Input: part model. Units: mm. Frame: model coordinates. A direction names the side the tool comes from. Coordinates: 2 decimals unless noted, no trailing zeros. Order: outer loops, then holes, each group sorted by start corner. A loop starts at its lowest first (then second) coordinate and runs counter-clockwise, first axis right, second up. Notation, with made-up numbers: (54, 50.25) - (84, 50.25) arc R18 ccw to (84, 60.25) - close; hole circle Ø4 at (-36.5, 0). An arc over 180 degrees is marked (long way). One line per question, with ' | ' between items.
Autodesk Inventor part; units mm, degrees
ref_plane "Work Plane2" through (5, 254.2, 0) normal (0, -1, 0) x (1, 0, 0)
ref_plane "Work Plane3" through (5, 144.2, 0) normal (0, -1, 0) x (1, 0, 0)
ref_plane "Work Plane4" through (0, 34.2, 0) normal (0, -1, 0) x (1, 0, 0)
sketch "Boceto1" plane through (0, 0, 0) normal (1, 0, 0) x (0, 1, 0)
  line L0 (0, 0) -> (330, 0)
  line L1 (330, 0) -> (330, -75)
  line L2 (330, -75) -> (0, -75)
  line L3 (0, -75) -> (0, 0)
  dimension "d0" = 330
  dimension "d1" = 75
extrude "Extrusión1" add sketch "Boceto1" along normal blind 5
sketch "Boceto2" plane through (5, 0, 0) normal (1, 0, 0) x (0, 0, -1)
  line L0 (75, 330) -> (0, 330)
  line L1 (75, 0) -> (75, 330)
  line L2 (0, 330) -> (75, 330)
  line L3 (75, 330) -> (75, 250)
  line L4 (75, 250) -> (0, 250)
  line L5 (0, 250) -> (0, 330)
  line L6 (75, 140) -> (0, 140)
  line L7 (0, 140) -> (0, 220)
  line L8 (0, 220) -> (75, 220)
  line L9 (75, 220) -> (75, 140)
  line L10 (75, 30) -> (0, 30)
  line L11 (0, 30) -> (0, 110)
  line L12 (0, 110) -> (75, 110)
  line L13 (75, 110) -> (75, 30)
  point P0 (0, 0)
  dimension "d4" = 80
  dimension "d7" = 110
extrude "Extrusión2" add sketch "Boceto2" along normal blind 4
sketch "Boceto3" plane through (0, 330, 0) normal (0, 1, 0) x (1, 0, 0)
  line L0 (7, 0) -> (4, 0)
  line L1 (4, 0) -> (4, 75)
  line L2 (4, 75) -> (7, 75)
  line L3 (7, 75) -> (7, 0)
  line L4 (0, 75) -> (0, 0)
  line L5 (9, 75) -> (9, 0)
  line L6 (0, 0) -> (9, 0)
  line L7 (0, 75) -> (9, 75)
  dimension "d14" = 4
  dimension "d15" = 2
  dimension "d16" = 0
  dimension "d17" = 0
  dimension "d62" = 3
sketch "Boceto8" plane through (5, 220, 0) normal (0, 1, 0) x (1, 0, 0)
  line L0 (-1, 0) -> (-1, 75)
  line L1 (2, 75) -> (2, 0)
  line L2 (-5, 0) -> (4, 0)
  line L3 (-5, 75) -> (4, 75)
sketch "Boceto9" plane through (5, 110, 0) normal (0, 1, 0) x (1, 0, 0)
  line L0 (2, 75) -> (2, 0)
  line L1 (-1, 0) -> (-1, 75)
  line L2 (-5, 0) -> (4, 0)
  line L3 (-5, 75) -> (4, 75)
extrude "Extrusión3" cut sketch "Boceto3" against normal blind 30 contours L0 L1 L2 L3
extrude "Extrusión4" cut sketch "Boceto8" against normal blind 30
extrude "Extrusión5" cut sketch "Boceto9" against normal blind 30
sketch "Boceto10" plane through (0, 0, 0) normal (-1, 0, 0) x (0, 0, 1)
  line L0 (-75, 0) -> (-75, 330)
  line L1 (-75, 330) -> (0, 330)
  line L2 (-75, 0) -> (-70, 0)
  line L3 (-70, 0) -> (-70, 330)
  line L4 (-70, 330) -> (-75, 330)
  line L5 (-75, 330) -> (-75, 0)
  point P0 (0, 0)
  dimension "d24" = 5
extrude "Extrusión6" add sketch "Boceto10" against normal blind 100
sketch "Boceto11" plane through (5, 0, -70) normal (0, 0, 1) x (1, 0, 0)
  line L0 (95, 330) -> (95, 0)
  line L1 (-5, 0) -> (95, 0)
  line L2 (95, 330) -> (90, 330)
  line L3 (90, 330) -> (90, 0)
  line L4 (90, 0) -> (95, 0)
  line L5 (95, 0) -> (95, 330)
  dimension "d27" = 5
extrude "Extrusión7" add sketch "Boceto11" along normal blind 70
sketch "Boceto12" plane through (95, 0, -70) normal (-1, 0, 0) x (0, 0, 1)
  line L0 (70, 0) -> (70, 330)
  line L1 (-5, 0) -> (-5, 330)
  line L2 (70, 250) -> (-5, 250)
  line L3 (-5, 250) -> (-5, 220)
  line L4 (-5, 220) -> (70, 220)
  line L5 (70, 220) -> (70, 250)
  line L6 (-5, 330) -> (70, 330)
  line L7 (70, 140) -> (-5, 140)
  line L8 (-5, 140) -> (-5, 110)
  line L9 (-5, 110) -> (70, 110)
  line L10 (70, 110) -> (70, 140)
  line L11 (70, 30) -> (-5, 30)
  line L12 (-5, 30) -> (-5, 0)
  line L13 (-5, 0) -> (70, 0)
  line L14 (70, 0) -> (70, 30)
  point P0 (70, 0)
  point P1 (70, 30)
  point P2 (-5, 30)
  point P3 (70, 140)
  point P4 (-5, 140)
  point P5 (-5, 250)
  dimension "d30" = 80
  dimension "d31" = 30
  dimension "d34" = 110
extrude "Extrusión8" add sketch "Boceto12" along normal blind 4 contours L13 L1 L11 L0 | L9 L1 L7 L0 | L4 L1 L2 L0
sketch "Boceto16" plane through (100, 0, 0) normal (1, 0, 0) x (0, 0, -1)
  line L0 (70, 250) -> (0, 250)
  line L1 (0, 330) -> (0, 250)
  line L2 (70, 330) -> (0, 330)
  line L3 (70, 250) -> (70, 330)
  line L4 (70, 140) -> (0, 140)
  line L5 (0, 220) -> (0, 140)
  line L6 (0, 220) -> (70, 220)
  line L7 (70, 140) -> (70, 220)
  line L8 (70, 30) -> (0, 30)
  line L9 (0, 110) -> (0, 30)
  line L10 (0, 110) -> (70, 110)
  line L11 (70, 30) -> (70, 110)
  point P0 (0, 0)
extrude "Extrusión12" cut sketch "Boceto16" against normal blind 10
sketch "Boceto25" plane through (0, 0, 0) normal (0, 0, 1) x (1, 0, 0)
  line L0 (7, 330) -> (7, 300) construction
  line L1 (7, 300) -> (7, 330) construction
  line L2 (7, 330) -> (125.2499, 220) construction
  line L3 (7, 330) -> (9, 328.1395)
  line L4 (9, 330) -> (9, 250)
  line L5 (7, 330) -> (9, 330)
  line L6 (8, 330) -> (7, 330)
  line L7 (7, 220) -> (9, 220)
  line L8 (7, 220) -> (9, 218.1395)
  line L9 (9, 220) -> (9, 140)
  line L10 (7, 220) -> (9.7315, 220) construction
  line L11 (9, 218.1395) -> (9, 220)
  line L12 (9, 220) -> (7, 220)
  line L13 (7, 110) -> (9, 110)
  line L14 (7, 110) -> (9, 108.1395)
  line L15 (9, 108.1395) -> (9, 110)
  line L16 (9, 110) -> (7, 110)
  point P0 (0, 0)
  dimension "d57" = 42.93
  dimension "d106" = 42.93
extrude "Extrusión13" cut sketch "Boceto25" against normal blind 70
sketch "Boceto26" plane through (5, 0, 0) normal (1, 0, 0) x (0, 0, -1)
  line L0 (70, 0) -> (70, 30)
  line L1 (70, 30) -> (0, 30)
  line L2 (0, 30) -> (0, 0)
  line L3 (0, 0) -> (70, 0)
extrude "Extrusión14" cut sketch "Boceto26" against normal blind 10
sketch "Boceto27" plane through (91, 220, -70) normal (0, -1, 0) x (1, 0, 0)
  line L0 (0, 0) -> (0, 70) construction
  line L1 (0, 70) -> (-37.4235, 70) construction
  circle A0 centre (-7.5, 70) radius 7.5
  line L2 (0, 50) -> (-7.5, 50)
  line L3 (-7.5, 50) -> (-7.5, 70)
  line L4 (-7.5, 70) -> (0, 70)
  line L5 (0, 70) -> (0, 50)
  circle A1 centre (-7.5, 70) radius 4
  point P0 (-91, 70)
  point P1 (-7.5, 62.5)
  dimension "d64" = 15
  dimension "d63" = 20
  dimension "d65" = 8
sketch "Boceto28" plane through (91, 110, -70) normal (0, -1, 0) x (1, 0, 0)
  line L0 (0, 50) -> (-7.5, 50)
  line L1 (-7.5, 50) -> (-7.5, 70)
  circle A0 centre (-7.5, 70) radius 7.5
  circle A1 centre (-7.5, 70) radius 4
  line L2 (0, 70) -> (-37.4235, 70) construction
  line L3 (0, 70) -> (0, 50)
  point P0 (-91, 70)
  point P1 (-7.5, 62.5)
sketch "Boceto29" plane through (0, 0, -75) normal (0, -1, 0) x (1, 0, 0)
  line L0 (91, 55) -> (83.5, 55)
  line L1 (83.5, 55) -> (83.5, 75)
  circle A0 centre (83.5, 75) radius 7.5
  circle A1 centre (83.5, 75) radius 4
  line L2 (83.5, 75) -> (91, 75)
  line L3 (91, 75) -> (91, 55)
  point P0 (0, 75)
  point P1 (83.5, 67.5)
extrude "Extrusión15" add sketch "Boceto27" against normal blind 8.4 contours L4 A1 L3 A0 | L5 L2 L3 A0 | A0 L3 A1 L4
extrude "Extrusión16" add sketch "Boceto28" against normal blind 8.4
extrude "Extrusión17" add sketch "Boceto29" against normal blind 8.4 contours L0 L1 A0 L3 | L2 A1 L1 A0 | A0 L1 A1 L2
sketch "Boceto30" plane through (91, 220, -70) normal (0, -1, 0) x (1, 0, 0)
  circle A0 centre (-7.5, 70) radius 4
  line L0 (0, 0) -> (-91, 0)
  line L1 (-91, 0) -> (-91, -5)
  line L2 (-91, -5) -> (9, -5)
  line L3 (9, -5) -> (9, 70)
  line L4 (9, 70) -> (0, 70)
  arc A1 (0, 70) -> (-7.5, 62.5) centre (-7.5, 70) ccw
  line L5 (-7.5, 62.5) -> (-7.5, 50)
  line L6 (-7.5, 50) -> (0, 50)
  line L7 (0, 0) -> (0, 50)
  line L8 (0, 50) -> (0, 70)
  point P0 (-91, 70)
sketch "Boceto31" plane through (91, 110, -70) normal (0, -1, 0) x (1, 0, 0)
  line L0 (0, 50) -> (0, 70)
  circle A0 centre (-7.5, 70) radius 4
  line L1 (9, 0) -> (0, 0)
  line L2 (9, 70) -> (9, 0)
  line L3 (0, 70) -> (9, 70)
  arc A1 (0, 70) -> (-7.5, 62.5) centre (-7.5, 70) ccw
  line L4 (-7.5, 62.5) -> (-7.5, 50)
  line L5 (-7.5, 50) -> (0, 50)
  line L6 (0, 0) -> (0, 50)
  point P0 (-91, 70)
sketch "Boceto32" plane through (0, 0, -75) normal (0, -1, 0) x (1, 0, 0)
  circle A0 centre (83.5, 75) radius 4
  line L0 (100, 5) -> (91, 5)
  line L1 (100, 75) -> (100, 5)
  line L2 (91, 75) -> (100, 75)
  arc A1 (91, 75) -> (83.5, 67.5) centre (83.5, 75) ccw
  line L3 (83.5, 67.5) -> (83.5, 55)
  line L4 (83.5, 55) -> (91, 55)
  line L5 (91, 5) -> (91, 55)
  line L6 (91, 55) -> (91, 75)
  point P0 (0, 75)
extrude "Extrusión18" cut sketch "Boceto32" against normal blind 4.2 contours L4 L3 A1 L6
extrude "Extrusión19" cut sketch "Boceto31" against normal blind 4.2 contours L5 L4 A1 L0
extrude "Extrusión20" cut sketch "Boceto30" against normal blind 4.2 contours L6 L5 A1 L8
thread "Rosca1"
ref_plane "Work Plane2" through (5, 254.2, 0) normal (0, -1, 0) x (1, 0, 0)
sketch "Sketch33" plane through (5, 254.2, 0) normal (0, -1, 0) x (1, 0, 0)
  line L0 (4, 0) -> (4, -20)
  line L1 (4, -20) -> (11.5, -20)
  line L2 (11.5, -20) -> (11.5, 0)
  line L3 (11.5, 0) -> (4, 0)
  circle A0 centre (11.5, 0) radius 4
  circle A1 centre (11.5, 0) radius 7.5
  point P0 (-5, 0)
  point P1 (4, 0)
  point P2 (11.5, -7.5)
  dimension "d81" = 20
  dimension "d82" = 7.5
  dimension "d83" = 20
  dimension "d84" = 8
  dimension "d85" = 15
extrude "Extrusion21" add sketch "Sketch33" against normal blind 4.2 contours A1 L2 L1 L0 | A1 L2 A0 L3 | L3 A0 L2 A1
ref_plane "Work Plane3" through (5, 144.2, 0) normal (0, -1, 0) x (1, 0, 0)
sketch "Sketch34" plane through (5, 144.2, 0) normal (0, -1, 0) x (1, 0, 0)
  line L0 (4, 0) -> (4, -20)
  line L1 (4, -20) -> (11.5, -20)
  line L2 (11.5, -20) -> (11.5, 0)
  line L3 (11.5, 0) -> (4, 0)
  circle A0 centre (11.5, 0) radius 4
  circle A1 centre (11.5, 0) radius 7.5
  point P0 (-5, 0)
  point P1 (11.5, -7.5)
  dimension "d89" = 20
  dimension "d90" = 7.5
  dimension "d91" = 20
  dimension "d92" = 8
  dimension "d93" = 15
extrude "Extrusion22" add sketch "Sketch34" against normal blind 4.2 contours A1 L2 L1 L0 | A1 L2 A0 L3 | L3 A0 L2 A1
ref_plane "Work Plane4" through (0, 34.2, 0) normal (0, -1, 0) x (1, 0, 0)
sketch "Sketch35" plane through (0, 34.2, 0) normal (0, -1, 0) x (1, 0, 0)
  line L0 (9, 0) -> (9, -20)
  line L1 (9, -20) -> (16.5, -20)
  line L2 (16.5, -20) -> (16.5, 0)
  line L3 (16.5, 0) -> (9, 0)
  circle A0 centre (16.5, 0) radius 4
  circle A1 centre (16.5, 0) radius 7.5
  point P0 (0, 0)
  point P1 (9, 0)
  point P2 (16.5, -7.5)
  dimension "d97" = 20
  dimension "d98" = 7.5
  dimension "d99" = 20
  dimension "d100" = 8
  dimension "d101" = 15
extrude "Extrusion23" add sketch "Sketch35" against normal blind 4.2 contours A1 L2 L1 L0 | A1 L2 A0 L3 | L3 A0 L2 A1
thread "Thread2"
sketch "Boceto13" plane through (95, 250, 0) normal (0, 1, 0) x (1, 0, 0)
  line L0 (5, 70) -> (-4, 70)
  line L1 (-4, 0) -> (5, 0)
  line L2 (-2, 70) -> (1, 70)
  line L3 (1, 70) -> (1, 0)
  line L4 (1, 0) -> (-2, 0)
  line L5 (-2, 0) -> (-2, 70)
  line L6 (-4, 0) -> (-4, 70)
  point P0 (-2, 0)
  point P1 (1, 70)
  dimension "d113" = 2
  dimension "d114" = 3
extrude "Extrusión24" cut sketch "Boceto13" against normal blind 20 contours L3 L1 L5 L0
pattern_linear "Patrón rectangular1" count 3 spacing 110 along (0, -1, 0) of "Extrusión24"
equation "\"d57\" = d106"
properties part number "Interior Der" material "Plástico PBT"
Item 1: Draft query along Z for faces 6 (the face through (5, 125, -35)), 7 (the face through (79.504, 6.271, 0.176)), 8 (the face through (96.4, 235.2, 0)). Return one class per face: released by +Z, released by -Z, zero draft, split by the parting line, or undercut.
Data:
face 6: zero draft | face 7: undercut | face 8: released by +Z
Item 2: Section C-C on x = 33. Return the cut outline in (y, z), and give its area (3 significant figures).
Data:
outline: (0, -75) - (330, -75) - (330, -70) - (0, -70) - close | area: 1,650 mm^2
Item 3: Section A-A on y = 92. Return the cut outline in (x, z), and give its area (3 significant figures).
Data:
outline: (0, -75) - (100, -75) - (100, -70) - (9, -70) - (9, 0) - (7, 0) - (7, -70) - (4, -70) - (4, 0) - (0, 0) - close | area: 920 mm^2
Item 4: Section B-B on z = -62.5. Count the separate pieces of the cut face and the enclosed holes in it, and give its area (3 significant figures).
Data:
separate pieces: 4 | enclosed holes: 0 | area: 2,810 mm^2
Item 5: Access query for faces 1 (the face through (4, 315, -35)), 2 (the face through (96.4, 15.2, 0)), 3 (the face through (85, 8.4, -6)), 4 (the face through (93, 20, -35)), 5 (the face through (15, 148.4, -6)). Directions: +Z, -Z, +X, -X, +Y, -Y. A direction counts if a zero-diameter tool reaches every point of the face in a straight line with its end or side. Return the directions, or none.
Data:
face 1: +Z, +Y | face 2: +Z, +X, +Y, -Y | face 3: +Z, -X | face 4: +Z | face 5: +Z, +X
Item 6: Ray query, line 1 (Y direction, x = 95, z = -12.5); line 2 (Y direction, x = 85.5, z = -9); line 3 (X direction, y = 243.5, z = -66). Return the intervals inside material, ascending.
Data:
line 1: 0 to 10, 110 to 120, 220 to 230 | line 2: 4.2 to 8.4, 114.2 to 118.4, 224.2 to 228.4 | line 3: 0 to 5, 91 to 93, 96 to 100
Item 7: Contact query for flat-ended pins moving along their axis: P1, Ø8, axis at x = 56.5, y = 173, coming from the +Z side; P2, Ø0.6, axis at x = 91.5, z = -35.5, coming from the +Y side; P3, Ø1, axis at y = 173.5, z = -52, coming from the -X side; P4, Ø7, axis at x = 95, y = 233, coming from the +Z side. Output: stop coordinate, or through.
Data:
P1: z = -70 | P2: y = 250 | P3: x = 0 | P4: z = 0
